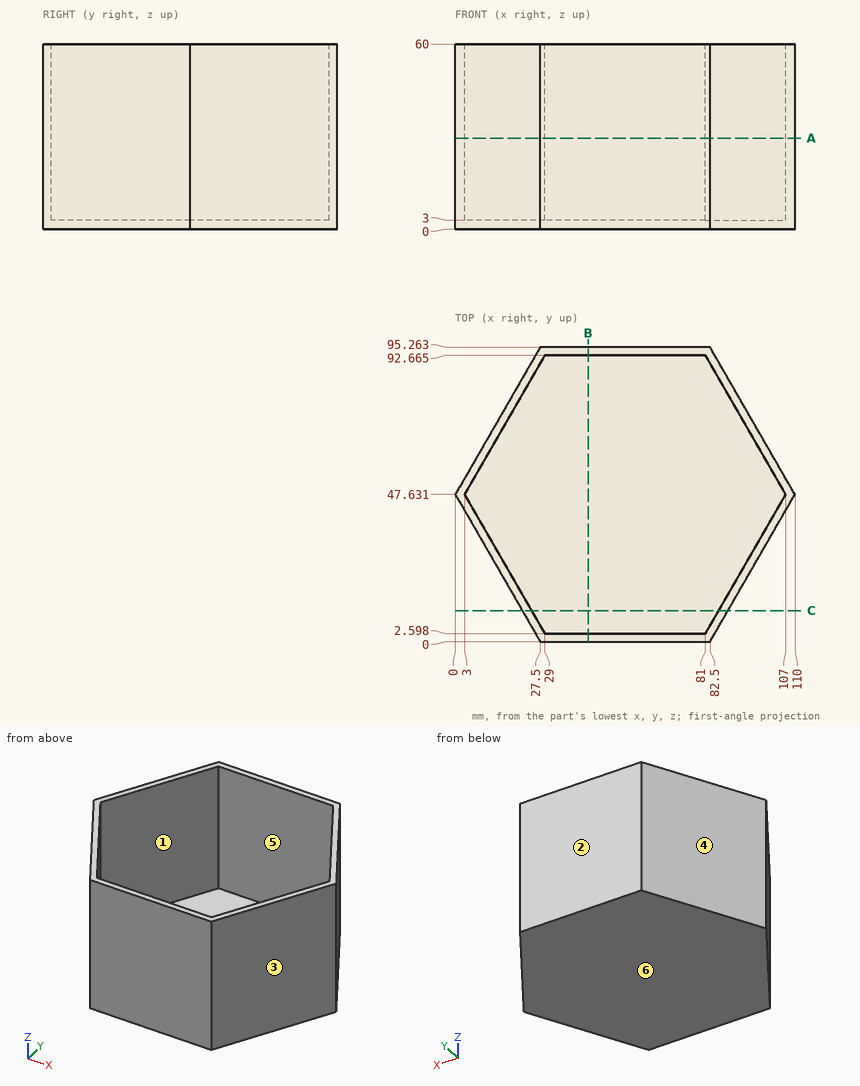
Study the drawing (mm; zero at the part's minimum x, y, z) and answer. A direction names the side the tool comes from. Give positions to 0.01 mm unless a question says otherwise; leave off trailing zeros. Order: outer loops, then holes, each group sorted by start corner. A loop starts at its lowest first (then second) coordinate and runs counter-clockwise, first axis right, second up. Notation, with made-up numbers: (-17.75, 59) - (1.25, 59) arc R12 ccw to (1.25, 63) - close; hole circle Ø9 at (59.5, -24). An arc over 180 degrees is marked (long way). Answer in a Markdown table with one row per item. Add a question column.
Q1. The part is cut by section A-A (z = 29.5). Determine the outline of the cut face in (x, y) (1 decimal).
Q2. Given P1, Ø10, axis at y = 16, z = 52.5, coming from the +X side (1 decimal); P2, Ø3, axis at x = 24.5, y = 19.5, coming from the +Z side; P3, Ø6, axis at x = 97.5, z = 9.5, coming from the +Y side, each flat-ended and moving along its own axis, determine where each tip first touches the part or whether it passes through.
Q3. The part is cut by section C-C (y = 10). Determine the outline of the cut face in (x, z).
Q4. The part is cut by section B-B (x = 43). Determine the outline of the cut face in (y, z) (1 decimal), then the cut area to 3 significant figures.
Q5. Find the intervals of material crossed by line 1 along Y through (x, z) = (36.5, 9) (1 decimal); line 2 along X through (y, z) = (60, 27); line 3 along X through (y, z) = (75, 21), in increasing order. Write a range as [from, to].
Q6. Which of the six approach directions +Z, -Z, +X, -X, +Y, -Y give full straight-line access (tool end or side, diameter ignored) to the marked faces 1 and 2?
Q7. For a pull along Y with two mould halves and no side action, classify the marked faces 3, 4, 5 and 6 as released by +Y, released by -Y, zero draft, split by the parting line, or undercut.
Determined:
| question | item | result |
|---|---|---|
| 1 | outline | (0, 47.6) - (27.5, 0) - (82.5, 0) - (110, 47.6) - (82.5, 95.3) - (27.5, 95.3) - close; hole (3, 47.6) - (29, 2.6) - (81, 2.6) - (107, 47.6) - (81, 92.7) - (29, 92.7) - close |
| 2 | P1 | stops at x = 94.6 |
| 2 | P2 | stops at z = 3 |
| 2 | P3 | stops at y = 74.48 |
| 3 | outline | (21.73, 0) - (88.27, 0) - (88.27, 60) - (85.27, 60) - (85.27, 3) - (24.73, 3) - (24.73, 60) - (21.73, 60) - close |
| 4 | outline | (0, 0) - (95.3, 0) - (95.3, 60) - (92.7, 60) - (92.7, 3) - (2.6, 3) - (2.6, 60) - (0, 60) - close |
| 4 | area | 582 mm² |
| 5 | line 1 | y = [0, 2.6], [92.7, 95.3] |
| 5 | line 2 | x = [7.14, 10.14], [99.86, 102.86] |
| 5 | line 3 | x = [15.8, 18.8], [91.2, 94.2] |
| 6 | face 1 | +Z |
| 6 | face 2 | +Z, -Z, +X, -X, +Y |
| 7 | face 3 | released by -Y |
| 7 | face 4 | released by +Y |
| 7 | face 5 | undercut |
| 7 | face 6 | zero draft |
